For this review, take the finished solid that the model builds, in its own axes (mm). A direction names the side the tool comes from. Round coordinates to 2 decimals unless told otherwise and drop trailing zeros. Order: outer loops, then holes, each group sorted by start corner. A loop starts at its lowest first (then second) coordinate and runs counter-clockwise, first axis right, second up. Notation, with made-up numbers: M -18,10 L 20,10 A35 ccw 20,42 Z; hole C -20,-24.5 d9. An arc over 180 degrees is marked long. Use a Markdown table: item, result.
from build123d import *

# Parameters (mm, degrees)
SKETCH1_W           = 2.54
SKETCH1_H           = 1.016
SKETCH1_W_2         = 5.08
BOSS_EXTRUDE1_DEPTH = 5.08
FILLET1_R           = 2.54
FILLET2_R           = 0.508


with BuildPart() as part:
    # Sketch1 → Boss-Extrude1 (new body)
    with BuildSketch(Plane.XY):
        with BuildLine():
            Line((-2.54, -4.399409051), (-2.54, -1.651))
            Line((-2.54, -1.651), (2.54, -1.651))
            Line((2.54, -1.651), (2.54, -4.399409051))
            ThreePointArc((2.54, -4.399409051), (4.399409051, -2.54), (5.08, 0))
            ThreePointArc((5.08, 0), (-2.54, 4.399409051), (-2.54, -4.399409051))
        make_face()
        with BuildLine():
            Line((2.54, -1.651), (-2.54, -1.651))
            Line((-2.54, -1.651), (-2.54, -4.399409051))
            ThreePointArc((-2.54, -4.399409051), (-1.314800749, -4.906903198), (0, -5.08))
            ThreePointArc((0, -5.08), (1.314800749, -4.906903198), (2.54, -4.399409051))
            Line((2.54, -4.399409051), (2.54, -1.651))
        make_face()
        with BuildLine():
            Line((-2.54, -4.399409051), (-2.54, -1.651))
            Line((-2.54, -1.651), (2.54, -1.651))
            Line((2.54, -1.651), (2.54, -4.399409051))
            ThreePointArc((2.54, -4.399409051), (4.399409051, -2.54), (5.08, 0))
            ThreePointArc((5.08, 0), (-2.54, 4.399409051), (-2.54, -4.399409051))
        make_face()
        with BuildLine():
            Line((2.54, -1.651), (-2.54, -1.651))
            Line((-2.54, -1.651), (-2.54, -4.399409051))
            ThreePointArc((-2.54, -4.399409051), (-1.314800749, -4.906903198), (0, -5.08))
            ThreePointArc((0, -5.08), (1.314800749, -4.906903198), (2.54, -4.399409051))
            Line((2.54, -4.399409051), (2.54, -1.651))
        make_face()
        with BuildLine():
            ThreePointArc((0, -5.08), (-1.314800749, -4.906903198), (-2.54, -4.399409051))
            Line((-2.54, -4.399409051), (-2.54, -5.08))
            Line((-2.54, -5.08), (0, -5.08))
        make_face()
        with BuildLine():
            Line((2.54, -5.08), (2.54, -4.399409051))
            ThreePointArc((2.54, -4.399409051), (1.314800749, -4.906903198), (0, -5.08))
            Line((0, -5.08), (2.54, -5.08))
        make_face()
        with Locations((1.27, -5.588)):
            Rectangle(SKETCH1_W, SKETCH1_H)
        with Locations((-5.08, -5.588)):
            Rectangle(SKETCH1_W_2, SKETCH1_H)
        with Locations((5.08, -5.588)):
            Rectangle(SKETCH1_W_2, SKETCH1_H)
        with Locations((-1.27, -5.588)):
            Rectangle(SKETCH1_W, SKETCH1_H)
    extrude(amount=BOSS_EXTRUDE1_DEPTH)

    # Fillet1
    # the kernel refuses this fillet: 2.54 mm, written as the material it adds along each edge
    with BuildSketch(Plane(origin=(-2.54, -5.08, 0), x_dir=(-1, 0, 0), z_dir=(0, 0, 1))) as fillet1_piece_1:
        with BuildLine():
            CenterArc((1.730375098, -2.54), FILLET1_R, 90, 42.941402865)
            Line((0, -0.680590949), (-0.034607502, -0.643402768))
            ThreePointArc((-0.034607502, -0.643402768), (-0.0508, -0.340295474), (-0.0508, 0))
            Line((-0.0508, 0), (0, 0.0508))
            Line((0, 0.0508), (1.730375098, 0.0508))
            Line((1.730375098, 0.0508), (1.730375098, 0))
        make_face()
    extrude(amount=5.08)
    with BuildSketch(Plane(origin=(2.54, -5.08, 0), x_dir=(0, 1, 0), z_dir=(0, 0, 1))) as fillet1_piece_2:
        with BuildLine():
            CenterArc((2.54, -1.730375098), FILLET1_R, 137.058597135, 42.941402865)
            Line((0, -1.730375098), (-0.0508, -1.730375098))
            Line((-0.0508, -1.730375098), (-0.0508, 0))
            Line((-0.0508, 0), (0, 0.0508))
            ThreePointArc((0, 0.0508), (0.340295474, 0.0508), (0.643402768, 0.034607502))
            Line((0.643402768, 0.034607502), (0.680590949, 0))
        make_face()
    extrude(amount=5.08)

    # Fillet2
    fillet2_edges = [part.edges().sort_by_distance(p)[0] for p in [
        (2.54, -4.399409051, 2.54),
        (-2.54, -4.399409051, 2.54),
    ]]
    fillet(fillet2_edges, radius=FILLET2_R)


solid = part.part
Q1. Add section B-B (y = -2). Write out the cut boundary in (x, z), then the cut area to 3 significant figures.
Determined:
| item | result |
|---|---|
| outline | M -4.67,0 L 4.67,0 L 4.67,5.08 L -4.67,5.08 Z |
| area | 47.4 mm^2 |
Q2. Machinability: for faces 4 (the cylindrical face through (-3.752, -5.027, 2.504)), 5 (the flat face through (0, 0, 5.08)), 6 (the cylindrical face through (3.737, -5.023, 2.504)), which of the approach directions +Z, -Z, +X, -X, +Y, -Y give a long, thin tool a straight path to every point of the face, cutting with its end or side? Answer none if there is none.
Determined:
| item | result |
|---|---|
| face 4 | +Z, -Z, -X |
| face 5 | +Z, +X, -X, +Y, -Y |
| face 6 | +Z, -Z, +X |
Q3. Draft analysis for pull direction Y (two halves, no side actions). For faces 1 (the flat face through (-6, -5.08, 3)), 2 (the flat face through (7.62, -5.6, 2.5)), 3 (the flat face through (0, -6.096, 3)), state which applies: pulls with the +Y half, pulls with the -Y half, needs draft (parallel to the pull), parting line crosses it, or undercut.
Determined:
| item | result |
|---|---|
| face 1 | undercut |
| face 2 | needs draft |
| face 3 | pulls with the -Y half |
Q4. Add section A-A (x = 3.75). Write out the cut boundary in (y, z).
Determined:
| item | result |
|---|---|
| outline | M -6.1,0 L -5.03,0 L -5.03,5.08 L -6.1,5.08 Z; M -3.43,0 L 3.43,0 L 3.43,5.08 L -3.43,5.08 Z |
Q5. Clearance check with flat-ended pins moving along their axes: pin 1 (1.7 mm diameter, centred on x = 6, z = 3.5, fed in from +Y); pin 2 (1 mm diameter, centred on y = -0.5, z = 4.5, fed in from +X). State where each tip first meets the part, or that it passes through.
Determined:
| item | result |
|---|---|
| pin 1 | stops at y = -5.08 |
| pin 2 | stops at x = 5.08 |
Q6. Add section C-C (y = 0.5). Write out the cut boundary in (x, z).
Determined:
| item | result |
|---|---|
| outline | M -5.06,0 L 5.06,0 L 5.06,5.08 L -5.06,5.08 Z |
Q7. Wall thickness on line 1 along Y through (x, z) = (3.75, 2.3); line 2 along Y through (x, z) = (4, 1); line 3 along Y through (x, z) = (-6, 3.75): over which ranges is each line inside the solid? List them lowest first. Write a range as [from, to].
Determined:
| item | result |
|---|---|
| line 1 | y = [-6.1, -5.03], [-3.43, 3.43] |
| line 2 | y = [-6.1, -5.07], [-3.13, 3.13] |
| line 3 | y = [-6.1, -5.08] |
